from build123d import *

# Parameters (mm, degrees)
SKETCH1_W                  = 38.1
SKETCH1_H                  = 44.45
SKETCH1_R                  = 13.081
BOSS_EXTRUDE1_DEPTH        = 12.7
F_4_40_TAPPED_HOLE1_D      = 2.2606
F_4_40_TAPPED_HOLE1_DEPTH  = 17.779
F_4_40_TAPPED_HOLE1_TIP    = 0.679152758
F_10_32_TAPPED_HOLE1_D     = 4.0386
F_10_32_TAPPED_HOLE1_DEPTH = 12.7
F_10_32_TAPPED_HOLE1_TIP   = 1.213317848


with BuildPart() as part:
    # Sketch1 → Boss-Extrude1 (new body)
    with BuildSketch(Plane.XY):
        with Locations((0, 22.225)):
            Rectangle(SKETCH1_W, SKETCH1_H)
        with Locations((0, 26.67)):
            Circle(SKETCH1_R, mode=Mode.SUBTRACT)
    extrude(amount=BOSS_EXTRUDE1_DEPTH)

    # #4-40 Tapped Hole1
    with Locations(Plane(origin=(0, 44.45, 0), x_dir=(-1, 0, 0), z_dir=(0, 1, 0))):
        with Locations((0, 6.35)):
            Hole(F_4_40_TAPPED_HOLE1_D / 2, depth=F_4_40_TAPPED_HOLE1_DEPTH)
            with Locations((0, 0, -(F_4_40_TAPPED_HOLE1_DEPTH + F_4_40_TAPPED_HOLE1_TIP / 2))):  # 118° drill point
                Cone(0, F_4_40_TAPPED_HOLE1_D / 2, F_4_40_TAPPED_HOLE1_TIP, mode=Mode.SUBTRACT)

    # #10-32 Tapped Hole1
    with Locations(Plane.XZ):
        with Locations((-12.7, 6.35), (12.7, 6.35)):
            Hole(F_10_32_TAPPED_HOLE1_D / 2, depth=F_10_32_TAPPED_HOLE1_DEPTH)
            with Locations((0, 0, -(F_10_32_TAPPED_HOLE1_DEPTH + F_10_32_TAPPED_HOLE1_TIP / 2))):  # 118° drill point
                Cone(0, F_10_32_TAPPED_HOLE1_D / 2, F_10_32_TAPPED_HOLE1_TIP, mode=Mode.SUBTRACT)


solid = part.part
Work out the finished part from the listing and answer in its coordinate system (mm). A direction names the side the tool comes from. Give positions to 0.01 mm unless a question says otherwise; leave off trailing zeros. Loops run counter-clockwise (first coordinate to the right, second up) from the corner with the lowest first, then second, coordinate; pieces in that order, holes last. Notation, with made-up numbers: M -16.75,-20.5 L 22.25,-20.5 A30 cw 22.25,3.5 Z; hole C 16.5,63 d3. An arc over 180 degrees is marked long. Use CSV: the item, a comma, the result in double quotes.
1) Determine the mould class of faces 4 (the conical face through (-12.366, 13.703, 6.455)), 5 (the flat face through (19.05, 22, 6)), 6 (the cylindrical face through (14.3, 6.44, 5.12)), 7 (the flat face through (0, 13, 0)) for opening direction Z: released by +Z, released by -Z, zero draft, split by the parting line, or undercut.
Answer:
face 4,"undercut"
face 5,"zero draft"
face 6,"undercut"
face 7,"released by -Z"
2) Find section A-A on x = 0. Write down the section's boundary in (y, z).
Answer:
outline,"M 0,0 L 13.59,0 L 13.59,12.7 L 0,12.7 Z; M 39.75,0 L 44.45,0 L 44.45,5.22 L 39.75,5.22 Z; M 39.75,7.48 L 44.45,7.48 L 44.45,12.7 L 39.75,12.7 Z"
3) Find section C-C on z = 1.5. Write down the section's boundary in (x, y).
Answer:
outline,"M -19.05,0 L 19.05,0 L 19.05,44.45 L -19.05,44.45 Z; hole C 0,26.67 d26.16"
4) Consider L1, parallel to X at y = 9.75, z = 6.35; L2, parallel to Y at x = 0, z = 4.5; L3, parallel to Z at x = -12.7, y = 4.75. Determine where each line is inside the solid, lowest interval first.
Answer:
L1,"-19.05 to -14.72, -10.68 to 10.68, 14.72 to 19.05"
L2,"0 to 13.59, 39.75 to 44.45"
L3,"0 to 4.33, 8.37 to 12.7"
5) Find section D-D on x = 4. Write down the section's boundary in (y, z).
Answer:
outline,"M 0,0 L 14.22,0 L 14.22,12.7 L 0,12.7 Z; M 39.12,0 L 44.45,0 L 44.45,12.7 L 39.12,12.7 Z"
6) Find section B-B on y = 26.67. Write down the section's boundary in (x, z).
Answer:
outline,"M -19.05,0 L -13.08,0 L -13.08,12.7 L -19.05,12.7 Z; M 13.08,0 L 19.05,0 L 19.05,12.7 L 13.08,12.7 Z"
7) Which of the six approach directions +Z, -Z, +X, -X, +Y, -Y give full straight-line access (tool end or side, diameter ignored) to faces 1 (the flat face through (-19.05, 22, 6)), 2 (the cylindrical face through (-11.1, 6.44, 5.12)), 3 (the cylindrical face through (-0.15, 42.04, 7.47))?
Answer:
face 1,"+Z, -Z, -X, +Y, -Y"
face 2,"-Y"
face 3,"+Y"
8) Given P1, Ø4, axis at x = -9, z = 9.5, coming from the -Y side; P2, Ø2.5, axis at x = -12.7, z = 6.35, coming from the -Y side; P3, Ø15.5, axis at x = 0, y = 26.67, coming from the -Z side; P4, Ø1.8, axis at x = 0, z = 6.35, coming from the +Y side, each flat-ended and moving along its own axis, determine where each tip first touches the part or whether it passes through.
Answer:
P1,"y = 0"
P2,"y = 13.16"
P3,"through"
P4,"y = 13.62"
